Geometry check sheet. Reference: the model listing, model coordinates, mm. A direction names the side the tool comes from. Coordinates: 2 decimals unless noted, no trailing zeros. Write each loop counter-clockwise with the first axis right and the second up, starting at its lowest first coordinate (ties: lowest second). Pieces come first, ordered by that corner, then holes. Notation, with made-up numbers: M 83,89 L 112,89 A22 cw 112,114 Z; hole C -13,-5.75 d1. An arc over 180 degrees is marked long. Write each question's results on one line, items separated by ' | '.
```python
from build123d import *

# Parameters (mm, degrees)
ESTRUSIONE_ESTRUSIONE1_DEPTH = 20
TAGLIO_ESTRUSIONE1_REACH     = 37.475
ESTRUSIONE_ESTRUSIONE4_DEPTH = 0.6
SCHIZZO12_W                  = 1.7
SCHIZZO12_H                  = 5.7
TAGLIO_ESTRUSIONE2_DEPTH     = 10


with BuildPart() as part:
    # Schizzo2 → Estrusione-Estrusione1 (new body)
    with BuildSketch(Plane.XY):
        with BuildLine():
            Line((-4, 9.5), (-10, 9.5))
            Line((-10, 9.5), (-10, 23.5))
            Line((-10, 23.5), (-5, 23.5))
            ThreePointArc((-5, 23.5), (-4.292893219, 23.207106781), (-4, 22.5))
            Line((-4, 22.5), (-4, 12.5))
            Line((-4, 12.5), (4, 12.5))
            Line((4, 12.5), (4, 9.5))
            Line((4, 9.5), (4, 6.5))
            Line((4, 6.5), (7.5, 6.5))
            Line((7.5, 6.5), (7.5, 4))
            Line((7.5, 4), (4, 0))
            Line((4, 0), (-4, 0))
            Line((-4, 0), (-7.5, 4))
            Line((-7.5, 4), (-7.5, 6.5))
            Line((-7.5, 6.5), (-4, 6.5))
            Line((-4, 6.5), (-4, 9.5))
        make_face()
    extrude(amount=-ESTRUSIONE_ESTRUSIONE1_DEPTH)

    # Schizzo6 → Taglio-Estrusione1 (cut, up to next)
    with BuildSketch(Plane.ZY.offset(10), mode=Mode.PRIVATE) as taglio_estrusione1_sk1:
        with BuildLine():
            Line((-8.5, 19.5), (-8.5, 17.5))
            ThreePointArc((-8.5, 17.5), (-10, 16), (-11.5, 17.5))
            Line((-11.5, 17.5), (-11.5, 19.5))
            ThreePointArc((-11.5, 19.5), (-10, 21), (-8.5, 19.5))
        make_face()
    taglio_estrusione1_tool1 = extrude(taglio_estrusione1_sk1.sketch, amount=-TAGLIO_ESTRUSIONE1_REACH, mode=Mode.PRIVATE) & part.part
    add(taglio_estrusione1_tool1.solids().sort_by_distance((-10, 18.5, -10))[0], mode=Mode.SUBTRACT)

    # Schizzo11 → Estrusione-Estrusione4 (add)
    with BuildSketch(Plane(origin=(0, 0, -20), x_dir=(-1, 0, 0), z_dir=(0, 0, -1))):
        Polygon((0.798177083, 7.666666667), (0.916666667, 7.666666667), (0.916666667, 3.166666667), (1.666666667, 3.166666667), (1.666666667, 2.5), (0.916666667, 2.5), (0.916666667, 1), (0.333333333, 1), (0.333333333, 2.5), (-2.75, 2.5), align=None)
        Polygon((0.333333333, 3.166666667), (0.333333333, 5.989583333), (-1.604166667, 3.166666667), align=None, mode=Mode.SUBTRACT)
    extrude(amount=ESTRUSIONE_ESTRUSIONE4_DEPTH)

    # Schizzo12 → Taglio-Estrusione2 (cut)
    with BuildSketch(Plane(origin=(0, 23.5, 0), x_dir=(1, 0, 0), z_dir=(0, 1, 0))):
        with Locations((-6.586432065, 10)):
            Rectangle(SCHIZZO12_W, SCHIZZO12_H)
    extrude(amount=-TAGLIO_ESTRUSIONE2_DEPTH, mode=Mode.SUBTRACT)


solid = part.part
```
Q1. Sectioned sample at C-C on z = -19. Record the cut outline in (x, y).
Geometry check:
outline: M -10,9.5 L -4,9.5 L -4,6.5 L -7.5,6.5 L -7.5,4 L -4,0 L 4,0 L 7.5,4 L 7.5,6.5 L 4,6.5 L 4,12.5 L -4,12.5 L -4,22.5 A1 ccw -5,23.5 L -10,23.5 Z
Q2. Sectioned sample at D-D on y = 11.25. Record the cut outline in (x, z), and give its area (3 significant figures).
Geometry check:
outline: M -10,-20 L 4,-20 L 4,0 L -10,0 Z | area: 280 mm2
Q3. Mould release check, pull along X, two halves, no side actions. Record for faces 6 (the flat face through (-9, 19, -8.5)), 7 (the flat face through (-7.436, 19, -8)), 8 (the flat face through (-7, 19, -7.15)), 9 (the flat face through (-4, 15, -10)): pulls with the +X half, pulls with the -X half, needs draft (parallel to the pull), parting line crosses it, or undercut.
Geometry check:
face 6: needs draft | face 7: undercut | face 8: undercut | face 9: pulls with the +X half
Q4. Scan lines: probe 1 along X at (y, z) = (15.5, -10.25); probe 2 along Y at (x, z) = (-5, -11); probe 3 along Z at (x, y) = (2, 1). Record each from-to range of solid material in increasing order.
Geometry check:
probe 1: x = -10 to -7.44, -5.74 to -4 | probe 2: y = 1.14 to 6.5, 9.5 to 16.38, 20.62 to 23.5 | probe 3: z = -20 to 0
Q5. Sectioned sample at B-B on x = -4.5. Record the cut outline in (y, z), and give its area (3 significant figures).
Geometry check:
outline: M 0.57,-20 L 6.5,-20 L 6.5,0 L 0.57,0 Z; M 9.5,-20 L 23.37,-20 L 23.37,0 L 9.5,0 Z; hole M 17.5,-11.5 L 19.5,-11.5 A1.5 ccw 19.5,-8.5 L 17.5,-8.5 A1.5 ccw Z | area: 383 mm2
Q6. Sectioned sample at A-A on z = -10. Record the cut outline in (x, y), and give its area (3 significant figures).
Geometry check:
outline: M -10,9.5 L -4,9.5 L -4,6.5 L -7.5,6.5 L -7.5,4 L -4,0 L 4,0 L 7.5,4 L 7.5,6.5 L 4,6.5 L 4,12.5 L -4,12.5 L -4,16 L -5.74,16 L -5.74,13.5 L -7.44,13.5 L -7.44,16 L -10,16 Z; M -10,21 L -7.44,21 L -7.44,23.5 L -10,23.5 Z; M -5.74,21 L -4,21 L -4,22.5 A1 ccw -5,23.5 L -5.74,23.5 Z | area: 177 mm2
Q7. Depth check by flat-ended pin: P1, Ø3, axis at y = 16.5, z = -8, coming from the +X side; P2, Ø9, axis at x = 1, z = -12, coming from the +Y side; P3, Ø2, axis at y = 5.5, z = -15, coming from the -X side. Enter the tip coordinate at first touch or a pass-through.
Geometry check:
P1: stops at x = -4 | P2: stops at y = 12.5 | P3: stops at x = -7.5
Q8. Access from +Z, -Z, +X, -X, +Y, -Y to the whole of each face (thin tool, end or side, straight path). Record for faces 1 (the flat face through (-3, 9, 0)), 2 (the flat face through (4, 10, -10)), 3 (the flat face through (-5, 18, -11.5)), 4 (the flat face through (-5.736, 19, -8)), 5 (the flat face through (-7, 9.5, -10)).
Geometry check:
face 1: +Z, +X, -X, +Y, -Y | face 2: +Z, -Z, +X, +Y | face 3: +X, -X | face 4: +Y | face 5: +Z, -Z, -X
